Read the model definition and answer for the solid it produces. Units are mm, in the model's axes. Face numbers are marked on the shaded views. A direction names the side the tool comes from. Round coordinates to 2 decimals unless told otherwise and drop trailing zeros. Loops run counter-clockwise (first coordinate to the right, second up) from the corner with the lowest first, then second, coordinate; pieces in that order, holes last. Notation, with made-up numbers: (18, 61) -> (47, 61) arc R25 ccw to (47, 99) -> close; hole circle Ø5 at (49, -6). An arc over 180 degrees is marked (long way). Put each result on its own line as item: value.
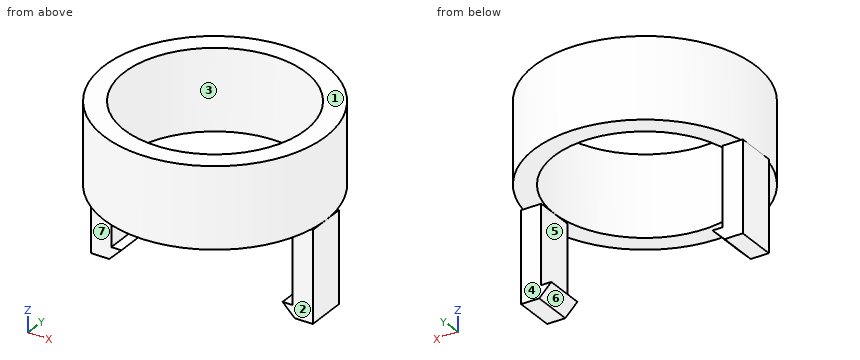
from build123d import *

# Parameters (mm, degrees)
SKETCH1_R           = 11
SKETCH1_R_2         = 9
BOSS_EXTRUDE1_DEPTH = 8
BOSS_EXTRUDE2_DEPTH = 2


with BuildPart() as part:
    # Sketch1 → Boss-Extrude1 (new body)
    with BuildSketch(Plane.XY):
        Circle(SKETCH1_R)
        Circle(SKETCH1_R_2, mode=Mode.SUBTRACT)
    extrude(amount=BOSS_EXTRUDE1_DEPTH)

    # Sketch2 → Boss-Extrude2 (add, symmetric)
    with BuildSketch(Plane(origin=(0, 0, 0), x_dir=(1, 0, 0), z_dir=(0, 1, 0))):
        Polygon((-11, 0), (-11, 9), (-9.2, 9), (-8, 7.8), (-9, 7.8), (-9, 0), align=None)
        Polygon((9, 0), (11, 0), (11, 9), (9.2, 9), (8, 7.8), (9, 7.8), align=None)
    extrude(amount=BOSS_EXTRUDE2_DEPTH, both=True)


solid = part.part
Item 1: Flat-ended cylindrical pins translate along their axes: pin 1 Ø10 at (y, z) = (-7.5, -7) entering from +X; pin 2 Ø8 at (x, y) = (-1.5, 8) entering from +Z; pin 3 Ø1.5 at (x, y) = (-5.5, -7.5) entering from -Z; pin 4 Ø3.5 at (x, z) = (9, -4) entering from +Y. Find the tip coordinate at first contact, or state that the pin passes through.
Derived:
pin 1: passes through
pin 2: stops at z = 8
pin 3: stops at z = 0
pin 4: stops at y = 2
Item 2: For a pull along Y with two mould halves and no side action, classify the marked faces 1, 2 and 3 as pulls with the +Y half, pulls with the -Y half, needs draft (parallel to the pull), parting line crosses it, or undercut.
Derived:
face 1: needs draft
face 2: pulls with the -Y half
face 3: undercut
Item 3: Find the intervals of material crossed by line 1 along X through (y, z) = (1.5, -5.25); line 2 along Y through (x, z) = (-5.75, 2), in increasing order.
Derived:
line 1: x = -11 to -9, 9 to 11
line 2: y = -9.38 to -6.92, 6.92 to 9.38
Item 4: The part is cut by section B-B (x = 0). Determine the outline of the cut face in (y, z), then the cut area to 3 significant figures.
Derived:
outline: (-11, 0) -> (-9, 0) -> (-9, 8) -> (-11, 8) -> close; (9, 0) -> (11, 0) -> (11, 8) -> (9, 8) -> close
area: 32.0 mm^2
Item 5: The part is cut by section D-D (z = 4). Determine the outline of the cut face in (x, y), then the cut area to 3 significant figures.
Derived:
outline: circle Ø22 at (0, 0); hole circle Ø18 at (0, 0)
area: 126 mm^2
Item 6: Which of the six approach directions +Z, -Z, +X, -X, +Y, -Y give full straight-line access (tool end or side, diameter ignored) to the marked faces 4, 5, 6 and 7?
Derived:
face 4: -Z, +X, -X, +Y
face 5: +Y, -Y
face 6: -Z, +Y, -Y
face 7: -Z, +X, -X, -Y
Item 7: The part is cut by section A-A (z = -2). Determine the outline of the cut face in (x, y), then the cut area to 3 significant figures.
Derived:
outline: (-11, -2) -> (-9, -2) -> (-9, 2) -> (-11, 2) -> close; (9, -2) -> (11, -2) -> (11, 2) -> (9, 2) -> close
area: 16.0 mm^2
